Read the model definition and answer for the solid it produces. Units are mm, in the model's axes. A direction names the side the tool comes from. Give positions to 0.01 mm unless a question says otherwise; leave off trailing zeros. Write each loop counter-clockwise with the first axis right and the second up, starting at its lowest first coordinate (ties: lowest second). Pieces come first, ordered by that corner, then holes. Notation, with made-up numbers: M 55.5,35 L 107.5,35 A17 ccw 107.5,44 Z; hole C 52,4.5 d7. An arc over 180 degrees is marked long. Answer as CSV lines item,"result". Start each with the question number.
```python
from build123d import *

# Parameters (mm, degrees)
ESQUISSE1_W               = 60
ESQUISSE1_H               = 54
ESQUISSE1_R               = 2
BOSS_EXTRU_1_DEPTH        = 2
ESQUISSE2_W               = 15
ESQUISSE2_H               = 13.5
BOSS_EXTRU_2_DEPTH        = 10
ENL_V_MAT_EXTRU_2_DEPTH   = 16
ESQUISSE5_W               = 4.75
ESQUISSE5_H               = 13.5
BOSS_EXTRU_3_DEPTH        = 12
ESQUISSE6_W               = 5.5
ESQUISSE6_H               = 8.66
ENL_V_MAT_EXTRU_3_DEPTH   = 6.25
ESQUISSE7_R               = 2.75
ENL_V_MAT_EXTRU_4_DEPTH   = 28
SYM_TRIE2_COPY_1_SKETCH_W = 15
SYM_TRIE2_COPY_1_SKETCH_H = 13.5
SYM_TRIE2_COPY_1_DEPTH    = 10
SYM_TRIE2_COPY_2_DEPTH    = 16
SYM_TRIE2_COPY_3_SKETCH_W = 4.75
SYM_TRIE2_COPY_3_SKETCH_H = 13.5
SYM_TRIE2_COPY_3_DEPTH    = 12
SYM_TRIE2_COPY_4_SKETCH_W = 5.5
SYM_TRIE2_COPY_4_SKETCH_H = 8.66
SYM_TRIE2_COPY_4_DEPTH    = 6.25
SYM_TRIE2_COPY_5_SKETCH_R = 2.75
SYM_TRIE2_COPY_5_DEPTH    = 28
ESQUISSE8_W               = 10.5
ESQUISSE8_H               = 3
BOSS_EXTRU_4_DEPTH        = 10
ESQUISSE12_W              = 15
ESQUISSE12_H              = 19
BOSS_EXTRU_6_DEPTH        = 10
ESQUISSE9_W               = 16.5
ESQUISSE9_H               = 16.5
ESQUISSE9_W_2             = 10.5
ESQUISSE9_H_2             = 10.5
BOSS_EXTRU_7_DEPTH        = 10
ENL_V_MAT_EXTRU_6_DEPTH   = 21
ESQUISSE13_W              = 10.5
ESQUISSE13_H              = 10.5
ENL_V_MAT_EXTRU_7_DEPTH   = 21
ESQUISSE15_R              = 2
ESQUISSE15_W              = 0.75
ESQUISSE15_H              = 2.25
BOSS_EXTRU_9_DEPTH        = 10
ENL_V_MAT_EXTRU_8_DEPTH   = 10
ESQUISSE17_W              = 10.5
ESQUISSE17_H              = 10.5
BOSS_EXTRU_10_DEPTH       = 5.5
ESQUISSE18_W              = 4.5
ESQUISSE18_H              = 4.330127019
ENL_V_MAT_EXTRU_9_DEPTH   = 1.5


with BuildPart() as part:
    # Esquisse1 → Boss.-Extru.1 (new body)
    with BuildSketch(Plane.XY):
        with Locations((30, -27)):
            Rectangle(ESQUISSE1_W, ESQUISSE1_H)
        with Locations((5, -27)):
            Circle(ESQUISSE1_R, mode=Mode.SUBTRACT)
        with Locations((30, -27)):
            Circle(ESQUISSE1_R, mode=Mode.SUBTRACT)
        with Locations((55, -27)):
            Circle(ESQUISSE1_R, mode=Mode.SUBTRACT)
    extrude(amount=BOSS_EXTRU_1_DEPTH)

    # Esquisse2 → Boss.-Extru.2 (add)
    with BuildSketch(Plane.XY.offset(2)):
        with Locations((7.5, -43.25)):
            Rectangle(ESQUISSE2_W, ESQUISSE2_H)
    boss_extru_2 = extrude(amount=BOSS_EXTRU_2_DEPTH)

    # Esquisse4 → Enlèv. mat.-Extru.2 (cut)
    with BuildSketch(Plane.ZY):
        Polygon((9.5, -45.415063509), (9.5, -41.084936491), (5.75, -38.919872981), (2, -41.084936491), (2, -45.415063509), (5.75, -47.580127019), align=None)
    enl_v_mat_extru_2 = extrude(amount=-ENL_V_MAT_EXTRU_2_DEPTH, mode=Mode.SUBTRACT)

    # Esquisse5 → Boss.-Extru.3 (add)
    with BuildSketch(Plane.XY.offset(12)):
        with Locations((2.375, -43.25)):
            Rectangle(ESQUISSE5_W, ESQUISSE5_H)
        with Locations((12.625, -43.25)):
            Rectangle(ESQUISSE5_W, ESQUISSE5_H)
    boss_extru_3 = extrude(amount=-BOSS_EXTRU_3_DEPTH)

    # Esquisse6 → Enlèv. mat.-Extru.3 (cut)
    with BuildSketch(Plane.XY.offset(12)):
        with Locations((7.5, -43.25)):
            Rectangle(ESQUISSE6_W, ESQUISSE6_H)
    enl_v_mat_extru_3 = extrude(amount=-ENL_V_MAT_EXTRU_3_DEPTH, mode=Mode.SUBTRACT)

    # Esquisse7 → Enlèv. mat.-Extru.4 (cut)
    with BuildSketch(Plane.ZY):
        with Locations((6.33, -43.25)):
            Circle(ESQUISSE7_R)
    enl_v_mat_extru_4 = extrude(amount=-ENL_V_MAT_EXTRU_4_DEPTH, mode=Mode.SUBTRACT)

    # Symétrie1: Boss.-Extru.2, Enlèv. mat.-Extru.2, Boss.-Extru.3, Enlèv. mat.-Extru.3, Enlèv. mat.-Extru.4 across plane
    add(boss_extru_2.mirror(Plane(origin=(0, -27, 0), x_dir=(0, 0, 1), z_dir=(0, -1, 0))))
    add(enl_v_mat_extru_2.mirror(Plane(origin=(0, -27, 0), x_dir=(0, 0, 1), z_dir=(0, -1, 0))), mode=Mode.SUBTRACT)
    add(boss_extru_3.mirror(Plane(origin=(0, -27, 0), x_dir=(0, 0, 1), z_dir=(0, -1, 0))))
    add(enl_v_mat_extru_3.mirror(Plane(origin=(0, -27, 0), x_dir=(0, 0, 1), z_dir=(0, -1, 0))), mode=Mode.SUBTRACT)
    add(enl_v_mat_extru_4.mirror(Plane(origin=(0, -27, 0), x_dir=(0, 0, 1), z_dir=(0, -1, 0))), mode=Mode.SUBTRACT)

    # Symétrie2: Boss.-Extru.2, Enlèv. mat.-Extru.2, Boss.-Extru.3, Enlèv. mat.-Extru.3, Enlèv. mat.-Extru.4 across plane
    add(boss_extru_2.mirror(Plane.ZY.offset(-30)))
    add(enl_v_mat_extru_2.mirror(Plane.ZY.offset(-30)), mode=Mode.SUBTRACT)
    add(boss_extru_3.mirror(Plane.ZY.offset(-30)))
    add(enl_v_mat_extru_3.mirror(Plane.ZY.offset(-30)), mode=Mode.SUBTRACT)
    add(enl_v_mat_extru_4.mirror(Plane.ZY.offset(-30)), mode=Mode.SUBTRACT)

    # Symétrie2 copy 1 sketch → Symétrie2 copy 1 (add)
    with BuildSketch(Plane(origin=(60, -54, 2), x_dir=(-1, 0, 0), z_dir=(0, 0, 1))):
        with Locations((7.5, -43.25)):
            Rectangle(SYM_TRIE2_COPY_1_SKETCH_W, SYM_TRIE2_COPY_1_SKETCH_H)
    extrude(amount=SYM_TRIE2_COPY_1_DEPTH)

    # Symétrie2 copy 2 sketch → Symétrie2 copy 2 (cut)
    with BuildSketch(Plane(origin=(60, -54, 0), x_dir=(0, 0, 1), z_dir=(1, 0, 0))):
        Polygon((9.5, -45.415063509), (9.5, -41.084936491), (5.75, -38.919872981), (2, -41.084936491), (2, -45.415063509), (5.75, -47.580127019), align=None)
    extrude(amount=-SYM_TRIE2_COPY_2_DEPTH, mode=Mode.SUBTRACT)

    # Symétrie2 copy 3 sketch → Symétrie2 copy 3 (add)
    with BuildSketch(Plane(origin=(60, -54, 12), x_dir=(-1, 0, 0), z_dir=(0, 0, 1))):
        with Locations((2.375, -43.25)):
            Rectangle(SYM_TRIE2_COPY_3_SKETCH_W, SYM_TRIE2_COPY_3_SKETCH_H)
        with Locations((12.625, -43.25)):
            Rectangle(SYM_TRIE2_COPY_3_SKETCH_W, SYM_TRIE2_COPY_3_SKETCH_H)
    extrude(amount=-SYM_TRIE2_COPY_3_DEPTH)

    # Symétrie2 copy 4 sketch → Symétrie2 copy 4 (cut)
    with BuildSketch(Plane(origin=(60, -54, 12), x_dir=(-1, 0, 0), z_dir=(0, 0, 1))):
        with Locations((7.5, -43.25)):
            Rectangle(SYM_TRIE2_COPY_4_SKETCH_W, SYM_TRIE2_COPY_4_SKETCH_H)
    extrude(amount=-SYM_TRIE2_COPY_4_DEPTH, mode=Mode.SUBTRACT)

    # Symétrie2 copy 5 sketch → Symétrie2 copy 5 (cut)
    with BuildSketch(Plane(origin=(60, -54, 0), x_dir=(0, 0, 1), z_dir=(1, 0, 0))):
        with Locations((6.33, -43.25)):
            Circle(SYM_TRIE2_COPY_5_SKETCH_R)
    extrude(amount=-SYM_TRIE2_COPY_5_DEPTH, mode=Mode.SUBTRACT)

    # Esquisse8 → Boss.-Extru.4 (add)
    with BuildSketch(Plane.XY.offset(2)):
        Polygon((35.25, -51), (35.25, -54), (38.25, -54), (38.25, -37.5), (21.75, -37.5), (21.75, -54), (24.75, -54), (24.75, -51), (24.75, -40.5), (35.25, -40.5), align=None)
        with Locations((30, -52.5)):
            Rectangle(ESQUISSE8_W, ESQUISSE8_H)
    boss_extru_4 = extrude(amount=BOSS_EXTRU_4_DEPTH)

    # Esquisse12 → Boss.-Extru.6 (add)
    with BuildSketch(Plane.XY.offset(2)):
        with Locations((7.5, -27)):
            Rectangle(ESQUISSE12_W, ESQUISSE12_H)
    boss_extru_6 = extrude(amount=BOSS_EXTRU_6_DEPTH)

    # Esquisse9 → Boss.-Extru.7 (add)
    with BuildSketch(Plane.XY.offset(2)):
        with Locations((14.25, -27)):
            Rectangle(ESQUISSE9_W, ESQUISSE9_H)
        with Locations((14.25, -27)):
            Rectangle(ESQUISSE9_W_2, ESQUISSE9_H_2, mode=Mode.SUBTRACT)
    boss_extru_7 = extrude(amount=BOSS_EXTRU_7_DEPTH)

    # Esquisse11 → Enlèv. mat.-Extru.6 (cut)
    with BuildSketch(Plane.XY.offset(2)):
        Polygon((8.935840957, -29.386947115), (8.935840957, -25.056820096), (5.185840957, -22.891756586), (1.435840957, -25.056820096), (1.435840957, -29.386947115), (5.185840957, -31.552010624), align=None)
    enl_v_mat_extru_6 = extrude(amount=ENL_V_MAT_EXTRU_6_DEPTH, mode=Mode.SUBTRACT)

    # Esquisse13 → Enlèv. mat.-Extru.7 (cut)
    with BuildSketch(Plane.XY.offset(2)):
        with Locations((14.25, -27)):
            Rectangle(ESQUISSE13_W, ESQUISSE13_H)
    enl_v_mat_extru_7 = extrude(amount=ENL_V_MAT_EXTRU_7_DEPTH, mode=Mode.SUBTRACT)

    # Symétrie3: Boss.-Extru.6, Boss.-Extru.7, Enlèv. mat.-Extru.6, Enlèv. mat.-Extru.7 across plane
    add(boss_extru_6.mirror(Plane.ZY.offset(-30)))
    add(boss_extru_7.mirror(Plane.ZY.offset(-30)))
    add(enl_v_mat_extru_6.mirror(Plane.ZY.offset(-30)), mode=Mode.SUBTRACT)
    add(enl_v_mat_extru_7.mirror(Plane.ZY.offset(-30)), mode=Mode.SUBTRACT)

    # Symétrie4: Boss.-Extru.4 across plane
    add(boss_extru_4.mirror(Plane(origin=(0, -27, 0), x_dir=(0, 0, 1), z_dir=(0, -1, 0))))

    # Esquisse15 → Boss.-Extru.9 (add)
    # profile 1 of 5: a face of its own
    with BuildSketch(Plane.XY.offset(2)):
        Polygon((22.5, -35.25), (22.5, -37.5), (37.5, -37.5), (37.5, -35.25), (37.5, -18.75), (37.5, -16.5), (22.5, -16.5), (22.5, -18.75), align=None)
        with Locations((30, -27)):
            Circle(ESQUISSE15_R, mode=Mode.SUBTRACT)
    # profile 2 of 5: a face of its own
    with BuildSketch(Plane.XY.offset(2)):
        with Locations((22.125, -36.375)):
            Rectangle(ESQUISSE15_W, ESQUISSE15_H)
    # profile 3 of 5: a face of its own
    with BuildSketch(Plane.XY.offset(2)):
        with Locations((37.875, -36.375)):
            Rectangle(ESQUISSE15_W, ESQUISSE15_H)
    # profile 4 of 5: a face of its own
    with BuildSketch(Plane.XY.offset(2)):
        with Locations((37.875, -17.625)):
            Rectangle(ESQUISSE15_W, ESQUISSE15_H)
    # profile 5 of 5: a face of its own
    with BuildSketch(Plane.XY.offset(2)):
        with Locations((22.125, -17.625)):
            Rectangle(ESQUISSE15_W, ESQUISSE15_H)
    extrude(amount=BOSS_EXTRU_9_DEPTH)

    # Esquisse16 → Enlèv. mat.-Extru.8 (cut)
    with BuildSketch(Plane.XY.offset(12)):
        Polygon((32.165063509, -23.25), (27.834936491, -23.25), (25.669872981, -27), (27.834936491, -30.75), (32.165063509, -30.75), (34.330127019, -27), align=None)
    extrude(amount=-ENL_V_MAT_EXTRU_8_DEPTH, mode=Mode.SUBTRACT)

    # Esquisse17 → Boss.-Extru.10 (add)
    with BuildSketch(Plane.XY.offset(2)):
        with Locations((14.25, -27)):
            Rectangle(ESQUISSE17_W, ESQUISSE17_H)
        with Locations((45.75, -27)):
            Rectangle(ESQUISSE17_W, ESQUISSE17_H)
        with Locations((30, -8.25)):
            Rectangle(ESQUISSE17_W, ESQUISSE17_H)
        with Locations((30, -45.75)):
            Rectangle(ESQUISSE17_W, ESQUISSE17_H)
    extrude(amount=BOSS_EXTRU_10_DEPTH)

    # Esquisse18 → Enlèv. mat.-Extru.9 (cut)
    with BuildSketch(Plane(origin=(9, 0, 0), x_dir=(0, 0, -1), z_dir=(1, 0, 0))):
        with Locations((-9.75, -27.221883606)):
            Rectangle(ESQUISSE18_W, ESQUISSE18_H)
    enl_v_mat_extru_9 = extrude(amount=-ENL_V_MAT_EXTRU_9_DEPTH, mode=Mode.SUBTRACT)

    # Symétrie5: Enlèv. mat.-Extru.9 across plane
    add(enl_v_mat_extru_9.mirror(Plane.ZY.offset(-30)), mode=Mode.SUBTRACT)


solid = part.part
```
1. Find section C-C on y = -10.75. State how many separate pieces and enclosed holes the cut face has, then the cut area to 3 significant figures.
2. Find the intervals of material crossed by line 1 (Y direction, x = 31.5, z = 10.75); line 2 (Y direction, x = 12.9, z = 6.33); line 3 (X direction, y = -36.5, z = 2.5), in increasing order. Write a range as [from, to].
3. Given pin 1 (3 mm diameter, centred on x = 5, z = 8, fed in from -Y); pin 2 (1.3 mm diameter, centred on x = 43.5, z = 10, fed in from -Y); pin 3 (6 mm diameter, centred on x = 47.5, z = 7, fed in from +Y), each flat-ended and moving along its own axis, determine where each tip first touches the part or whether it passes through.
4. Find section B-B on x = 13. Determine the outline of the cut face in (y, z), then the cut area to 3 significant figures.
5. Find section A-A on x = 30. Determine the outline of the cut face in (y, z).
6. Determine the mould class of faces 4 (the face through (30, -13.5, 10)), 5 (the face through (30, -8, 7.5)) for opening direction Z: +Z half, -Z half, draft (parallel to the pull), parting line (faces both ways), or undercut.
7. For faces 1 (the face through (42, -18.75, 7)), 2 (the face through (7.035, -30.485, 6.93)), 3 (the face through (21.75, -44, 7)), determine the directions among +Z, -Z, +X, -X, +Y, -Y from which every point of the face is accessible in a straight line to the end or side of a thin tool.
Computed:
1,separate pieces,"5"
1,enclosed holes,"0"
1,area,"323 mm^2"
2,line 1,"y = [-54, -51], [-40.5, -30.75], [-23.25, -13.5], [-3, 0]"
2,line 2,"y = [-50, -46], [-40.5, -13.5], [-8, -4]"
2,line 3,"x = [0, 15], [21.75, 38.25], [45, 60]"
3,pin 1,"stops at y = -50"
3,pin 2,"stops at y = -35.25"
3,pin 3,"stops at y = -4"
4,outline,"M -54,0 L 0,0 L 0,2 L -4,2 L -4,12 L -21.75,12 L -21.75,7.5 L -32.25,7.5 L -32.25,12 L -50,12 L -50,2 L -54,2 Z; hole C -43.25,6.33 d5.5; hole C -10.75,6.33 d5.5"
4,area,"473 mm^2"
5,outline,"M -54,0 L -29,0 L -29,2 L -30.75,2 L -30.75,12 L -40.5,12 L -40.5,7.5 L -51,7.5 L -51,12 L -54,12 Z; M -25,0 L 0,0 L 0,12 L -3,12 L -3,7.5 L -13.5,7.5 L -13.5,12 L -23.25,12 L -23.25,2 L -25,2 Z"
6,face 4,"draft"
6,face 5,"+Z half"
7,face 1,"+Z, +Y"
7,face 2,"+Z"
7,face 3,"+Z, -Y"
